from build123d import *

# Parameters (mm, degrees)
SKETCH1_R           = 5
BOSS_EXTRUDE1_DEPTH = 20
SKETCH2_R           = 2.27
CUT_EXTRUDE1_DEPTH  = 5.68
CUT_EXTRUDE1_TAPER  = 3.074
SKETCH7_R           = 1
CUT_EXTRUDE2_DEPTH  = 21
SKETCH9_R           = 2.27
CUT_EXTRUDE3_DEPTH  = 5.68
CUT_EXTRUDE3_TAPER  = 3.074


with BuildPart() as part:
    # Sketch1 → Boss-Extrude1 (new body)
    with BuildSketch(Plane.XY):
        Circle(SKETCH1_R)
    extrude(amount=BOSS_EXTRUDE1_DEPTH)

    # Sketch2 → Cut-Extrude1 (cut)
    with BuildSketch(Plane.XY):
        Circle(SKETCH2_R)
    extrude(amount=CUT_EXTRUDE1_DEPTH, taper=CUT_EXTRUDE1_TAPER, mode=Mode.SUBTRACT)

    # Sketch7 → Cut-Extrude2 (cut, through all)
    with BuildSketch(Plane.XY):
        Circle(SKETCH7_R)
    extrude(amount=CUT_EXTRUDE2_DEPTH, mode=Mode.SUBTRACT)

    # Sketch9 → Cut-Extrude3 (cut)
    with BuildSketch(Plane.XY.offset(20)):
        Circle(SKETCH9_R)
    extrude(amount=-CUT_EXTRUDE3_DEPTH, taper=CUT_EXTRUDE3_TAPER, mode=Mode.SUBTRACT)


solid = part.part
Design review of the part built by this model. Coordinates are the model's own, in mm. A direction names the side the tool comes from. Give positions to 0.01 mm unless a question says otherwise; leave off trailing zeros. Loops run counter-clockwise (first coordinate to the right, second up) from the corner with the lowest first, then second, coordinate; pieces in that order, holes last. Notation, with made-up numbers: M -34,70 L 13,70 A6 cw 13,79 Z; hole C -38.75,79.25 d3. An arc over 180 degrees is marked long. Answer as a JSON object with one key per item and string values.
Item 1: We need section B-B (z = 13.75). State the section outline as (x, y) points, and give its area (3 significant figures).
Output values:
{"outline": "C 0,0 d10; hole C 0,0 d2", "area": "75.4 mm2"}
Item 2: Wall thickness on line 1 along Y through (x, z) = (0, 10.5); line 2 along Z through (x, y) = (-0.75, 1.25); line 3 along X through (y, z) = (1.5, 3.25): over which ranges is each line inside the solid? List them lowest first.
Output values:
{"line 1": "y = -5 to -1, 1 to 5", "line 2": "z = 5.68 to 14.32", "line 3": "x = -4.77 to -1.46, 1.46 to 4.77"}
Item 3: We need section D-D (z = 16.75). State the section outline as (x, y) points.
Output values:
{"outline": "C 0,0 d10; hole C 0,0 d4.19"}
Item 4: We need section C-C (x = 2.75). State the section outline as (y, z) points.
Output values:
{"outline": "M -4.18,0 L 4.18,0 L 4.18,20 L -4.18,20 Z"}
Item 5: For P1, Ø3, axis at x = 0, y = 0, coming from the +Z side; P2, Ø1.5, axis at x = -3.5, y = 1.5, coming from the -Z side; P3, Ø4, axis at x = -3, z = 10, coming from the -Y side, all flat-tipped, find the tip position at first contact; note any pin that passes through.
Output values:
{"P1": "stops at z = 14.32", "P2": "stops at z = 0", "P3": "stops at y = -4.9"}
Item 6: Mouldability with a two-part tool opening along Y and no side actions: class faces 3 (the face through (-1.08, -4.88, 9.86)), 4 (the face through (1, -1, 14.32)), 5 (the face through (2.2, 1.2, 0)) as pulls with the +Y half, pulls with the -Y half, needs draft (parallel to the pull), parting line crosses it, or undercut.
Output values:
{"face 3": "parting line crosses it", "face 4": "undercut", "face 5": "needs draft"}
Item 7: Machinability: for faces 1 (the face through (1, -1, 5.68)), 2 (the face through (2.018, 0.635, 17.12)), which of the approach directions +Z, -Z, +X, -X, +Y, -Y give a long, thin tool a straight path to every point of the face, cutting with its end or side? Answer none if there is none.
Output values:
{"face 1": "-Z", "face 2": "+Z"}
Item 8: We need section A-A (x = 0). State the section outline as (y, z) points.
Output values:
{"outline": "M -5,0 L -2.27,0 L -1.96,5.68 L -1,5.68 L -1,14.32 L -1.96,14.32 L -2.27,20 L -5,20 Z; M 1,5.68 L 1.96,5.68 L 2.27,0 L 5,0 L 5,20 L 2.27,20 L 1.96,14.32 L 1,14.32 Z"}
